Here's the drawing with two shaded views (mm, measured from the low corner). I have some questions. A direction names the side the tool comes from. Coordinates: 2 decimals unless noted, no trailing zeros. Write each loop counter-clockwise with the first axis right and the second up, starting at its lowest first coordinate (ties: lowest second). Pieces come first, ordered by that corner, then holes.
Item 1: If we section it at A-A (x = 63.5): Please give me the cut outline in (y, z).
Item 2: If we section it at D-D (z = 26): Please give me the cut outline in (x, y).
Item 3: For the marked faces 1 and 2, which set-ups out of +Z, -Z, +X, -X, +Y, -Y let a thin tool reach every point of the face, with its end or its side?
Item 4: We'd pull the mould along X, two halves only. Please class the marked faces 3 and 4: +X half, -X half, draft (parallel to the pull), parting line (faces both ways), or undercut.
Item 5: I'm going to push flat-ended pins straight in: pin 1 Ø14 at (y, z) = (34.5, 24) entering from +X; pin 2 Ø3.5 at (y, z) = (7.5, 19) entering from -X; pin 3 Ø8 at (x, y) = (115, 5) entering from -Z. Where does each tip first touch, or does it pass through?
Item 6: If I drill on line 1 (Y direction, x = 5, z = 46); line 2 (Y direction, x = 81.5, z = 43.5); line 3 (X direction, y = 24, z = 46), over which ranges is the centre line in solid material (lowest first)?
Item 7: If we section it at B-B (y = 34): Please give me the cut outline in (x, z), then the cut area to 3 significant figures.
Item 8: If we section it at C-C (x = 5): Please give me the cut outline in (y, z).
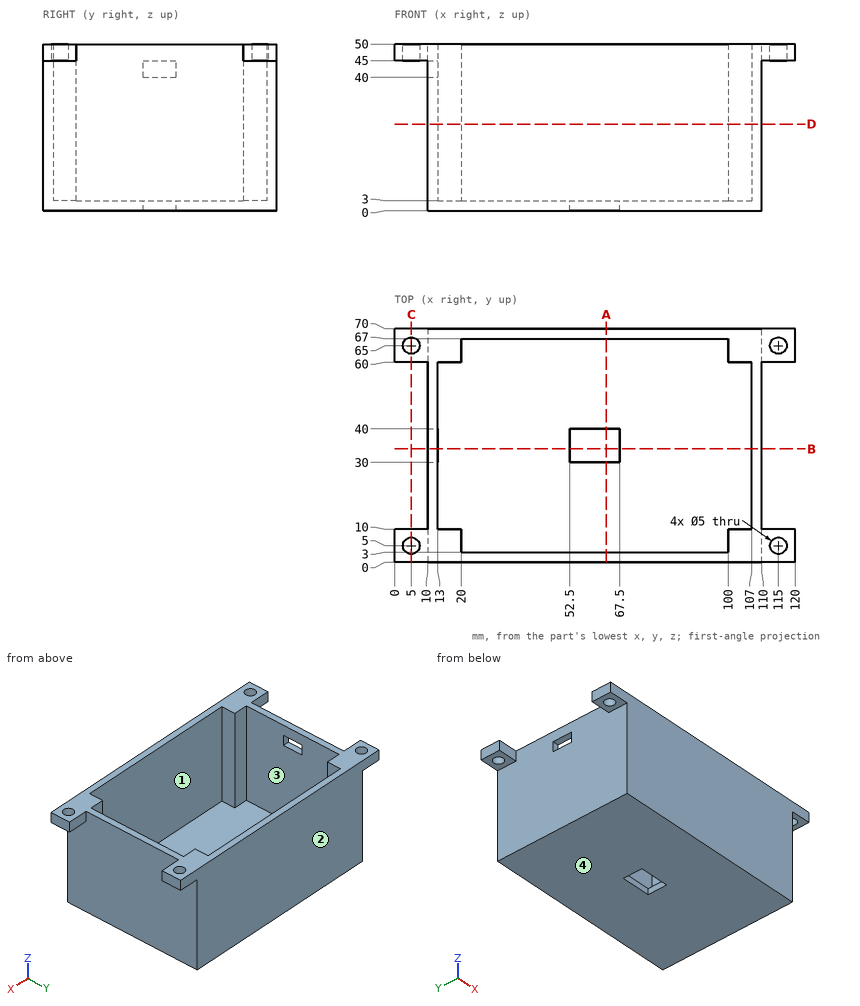
Answer list:
1. outline: (0, 0) - (30, 0) - (30, 3) - (3, 3) - (3, 50) - (0, 50) - close; (40, 0) - (70, 0) - (70, 50) - (67, 50) - (67, 3) - (40, 3) - close
2. outline: (10, 0) - (110, 0) - (110, 70) - (10, 70) - close; hole (13, 10) - (20, 10) - (20, 3) - (100, 3) - (100, 10) - (107, 10) - (107, 60) - (100, 60) - (100, 67) - (20, 67) - (20, 60) - (13, 60) - close
3. face 1: +Z
3. face 2: +Z, -Z, +X, -X, +Y
4. face 3: undercut
4. face 4: draft
5. pin 1: stops at x = 110
5. pin 2: stops at x = 10
5. pin 3: stops at z = 45
6. line 1: y = 0 to 2.5, 7.5 to 10, 60 to 62.5, 67.5 to 70
6. line 2: y = 0 to 3, 67 to 70
6. line 3: x = 10 to 13, 107 to 110
7. outline: (10, 0) - (52.5, 0) - (52.5, 3) - (13, 3) - (13, 40) - (10, 40) - close; (10, 45) - (13, 45) - (13, 50) - (10, 50) - close; (67.5, 0) - (110, 0) - (110, 50) - (107, 50) - (107, 3) - (67.5, 3) - close
7. area: 522 mm2
8. outline: (0, 45) - (2.5, 45) - (2.5, 50) - (0, 50) - close; (7.5, 45) - (10, 45) - (10, 50) - (7.5, 50) - close; (60, 45) - (62.5, 45) - (62.5, 50) - (60, 50) - close; (67.5, 45) - (70, 45) - (70, 50) - (67.5, 50) - close
